Can you work these out from the model? Positions are in its coordinate system, mm. A direction names the side the tool comes from. Coordinates: 2 decimals unless noted, no trailing zeros. Write each loop counter-clockwise with the first axis right and the second up, starting at its lowest first coordinate (ties: lowest second). Pieces come first, ordered by that corner, then holes.
```python
from build123d import *

# Parameters (mm, degrees)
SKETCH3_R          = 3.96875
CUT_EXTRUDE1_DEPTH = 12.7
CIRPATTERN2_COUNT  = 2


with BuildPart() as part:
    # Sketch1 → Revolve1 (revolve)
    with BuildSketch(Plane.XY, mode=Mode.PRIVATE) as revolve1_sk:
        Polygon((0, 0), (88.9, 0), (88.9, 31.75), (95.25, 31.75), (95.25, 76.2), (0, 76.2), align=None)
    revolve(revolve1_sk.sketch.rotate(Axis((0, 0, 0), (0, 1, 0)), 90), axis=Axis((0, 0, 0), (0, 1, 0)))

    # Sketch3 → Cut-Extrude1 (cut)
    with BuildSketch(Plane(origin=(88.9, 0, 0), x_dir=(0, 0, -1), z_dir=(1, 0, 0))):
        with Locations((0, 12.7)):
            Circle(SKETCH3_R)
    cut_extrude1 = extrude(amount=-CUT_EXTRUDE1_DEPTH, mode=Mode.SUBTRACT)

    # CirPattern2: Cut-Extrude1 ×2 about axis
    cirpattern2_axis = Axis((0, 0, 0), (0, -1, 0))
    for i in range(1, CIRPATTERN2_COUNT):
        add(cut_extrude1.rotate(cirpattern2_axis, i * 360 / CIRPATTERN2_COUNT), mode=Mode.SUBTRACT)


solid = part.part
```
1. If we section it at C-C, the plane x = 0: List the corners of the cut face in (y, z) for me, plus the area to 3 significant figures.
2. I'm going to push flat-ended pins straight in: P1, Ø6.5, axis at y = 11.5, z = -2, coming from the +X side; P2, Ø4, axis at x = 36, y = 28.5, coming from the -Z side; P3, Ø5, axis at y = 12.7, z = 0, coming from the -X side. Where does each tip first touch, or does it pass through?
3. If we section it at D-D, the plane y = 43: List the corners of the cut face in (x, z) for me.
4. If I drill on L1, parallel to Y at x = -86, z = 0; L2, parallel to Y at x = -66, z = 60; L3, parallel to Z at x = -79, y = 12, over which ranges is the centre line in solid material (lowest first)?
5. Which directions (+Z, -Z, +X, -X, +Y, -Y) give clear straight access to the entire face, cutting with the end or side of a thin tool? Please do faces 1 (the face through (82.639, 8.826, 0.86)), 2 (the face through (-1, 0, -1)), 3 (the face through (-60.083, 16.097, 65.523)), 4 (the face through (-82.64, 9.18, 1.83)).
6. If we section it at A-A, the plane z = 0: List the corners of the cut face in (x, y) for me, plus the area to 3 significant figures.
7. If we section it at B-B, the plane y = 12.7: List the corners of the cut face in (x, z) for me.
Answers:
1. outline: (0, -88.9) - (31.75, -88.9) - (31.75, -95.25) - (76.2, -95.25) - (76.2, 95.25) - (31.75, 95.25) - (31.75, 88.9) - (0, 88.9) - close
1. area: 14,100 mm2
2. P1: stops at x = 88.9
2. P2: stops at z = -82.14
2. P3: stops at x = -76.2
3. outline: circle Ø190.5 at (0, 0)
4. L1: y = 0 to 8.73, 16.67 to 76.2
4. L2: y = 31.75 to 76.2
4. L3: z = -40.77 to -3.91, 3.91 to 40.77
5. face 1: +X
5. face 2: +Z, -Z, +X, -X, -Y
5. face 3: -Y
5. face 4: -X
6. outline: (-95.25, 31.75) - (-88.9, 31.75) - (-88.9, 16.67) - (-76.2, 16.67) - (-76.2, 8.73) - (-88.9, 8.73) - (-88.9, 0) - (88.9, 0) - (88.9, 8.73) - (76.2, 8.73) - (76.2, 16.67) - (88.9, 16.67) - (88.9, 31.75) - (95.25, 31.75) - (95.25, 76.2) - (-95.25, 76.2) - close
6. area: 13,900 mm2
7. outline: (-88.81, -3.97) arc R88.9 ccw to (88.81, -3.97) - (76.2, -3.97) - (76.2, 3.97) - (88.81, 3.97) arc R88.9 ccw to (-88.81, 3.97) - (-76.2, 3.97) - (-76.2, -3.97) - close
